Design review of the part shown in the three views and the two pictorial views. Dimensions are in mm from the part's minimum x, y and z. A direction names the side the tool comes from. Coordinates: 2 decimals unless noted, no trailing zeros. Loops run counter-clockwise (first coordinate to the right, second up) from the corner with the lowest first, then second, coordinate; pieces in that order, holes last. Notation, with made-up numbers: (37.25, 14) -> (54.25, 14) arc R27 ccw to (54.25, 52) -> close; hole circle Ø5 at (85, 69.25). An arc over 180 degrees is marked (long way). Answer in a Markdown table with one row per item.
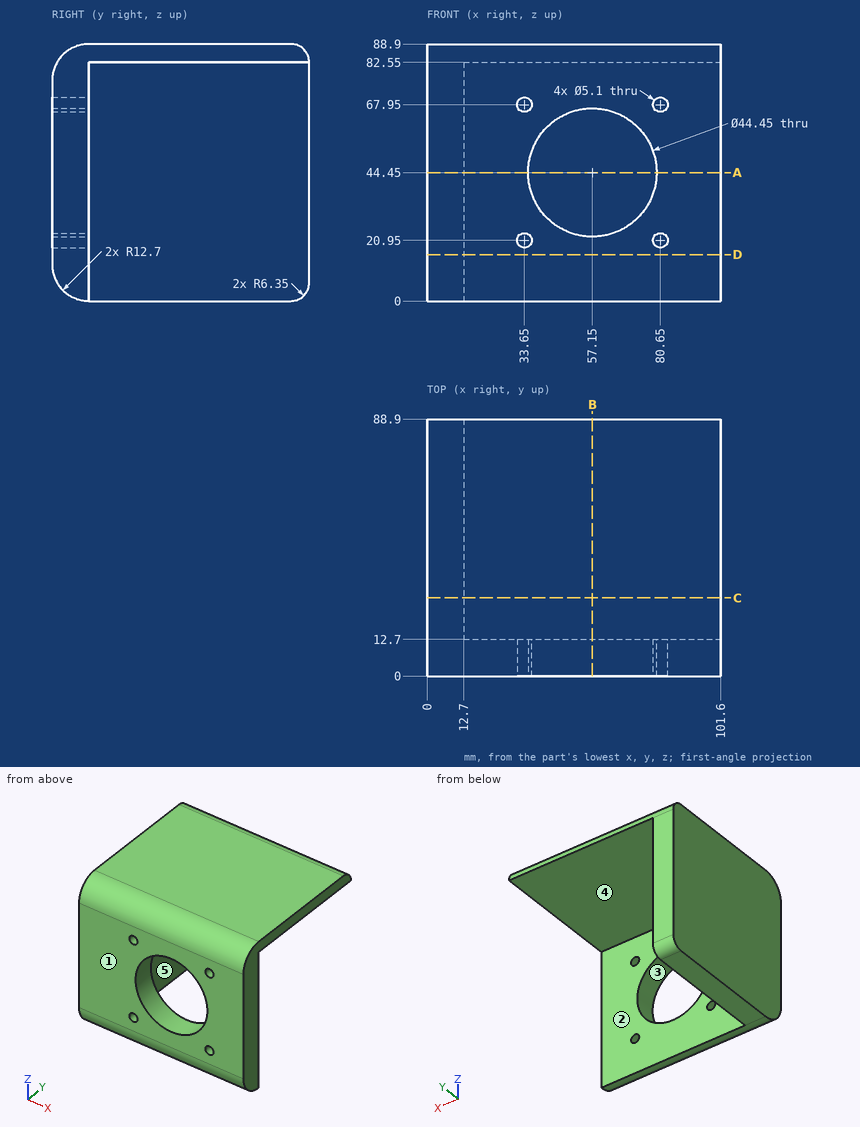
(1) Take a section at D-D on z = 16. Give the boundary of the cut face in (x, y).
Evaluation:
| item | result |
|---|---|
| outline | (0, 0) -> (101.6, 0) -> (101.6, 12.7) -> (12.7, 12.7) -> (12.7, 88.9) -> (0, 88.9) -> close |
(2) Take a section at C-C on y = 27. Give the boundary of the cut face in (x, z), and give its area (3 significant figures).
Evaluation:
| item | result |
|---|---|
| outline | (0, 0) -> (12.7, 0) -> (12.7, 82.55) -> (101.6, 82.55) -> (101.6, 88.9) -> (0, 88.9) -> close |
| area | 1,690 mm² |
(3) Tool access review of the marked faces 1 and 2: name each direction out of +Z, -Z, +X, -X, +Y, -Y from which nothing blocks a thin tool from reaching the whole face with its end or side.
Evaluation:
| item | result |
|---|---|
| face 1 | +Z, -Z, +X, -X, -Y |
| face 2 | -Z, +X, +Y |
(4) For pin 1 (6 mm diameter, centred on x = 38.5, z = 72.5, fed in from +Y); pin 2 (23 mm diameter, centred on y = 36.5, z = 55.5, fed in from +X); pin 3 (2 mm diameter, centred on x = 18, y = 77, fed in from -Z); pin 4 (4.5 mm diameter, centred on x = 80.65, z = 20.95, fed in from +Y), all flat-tipped, find the tip position at first contact; note any pin that passes through.
Evaluation:
| item | result |
|---|---|
| pin 1 | stops at y = 12.7 |
| pin 2 | stops at x = 12.7 |
| pin 3 | stops at z = 82.55 |
| pin 4 | passes through |
(5) Draft analysis for pull direction X (two halves, no side actions). For the marked faces 3, 4 and 5, state which applies: pulls with the +X half, pulls with the -X half, needs draft (parallel to the pull), parting line crosses it, or undercut.
Evaluation:
| item | result |
|---|---|
| face 3 | undercut |
| face 4 | needs draft |
| face 5 | pulls with the +X half |
(6) Take a section at A-A on z = 44.45. Give the boundary of the cut face in (x, y) (3 decimals).
Evaluation:
| item | result |
|---|---|
| outline | (0, 0) -> (34.925, 0) -> (34.925, 12.7) -> (12.7, 12.7) -> (12.7, 88.9) -> (0, 88.9) -> close; (79.375, 0) -> (101.6, 0) -> (101.6, 12.7) -> (79.375, 12.7) -> close |
(7) Take a section at B-B on x = 57.15. Give the boundary of the cut face in (y, z) (3 decimals), and give its area (3 significant figures).
Evaluation:
| item | result |
|---|---|
| outline | (0, 12.7) arc R12.7 ccw to (12.7, 0) -> (12.7, 22.225) -> (0, 22.225) -> close; (0, 66.675) -> (12.7, 66.675) -> (12.7, 82.55) -> (88.9, 82.55) arc R6.35 ccw to (82.55, 88.9) -> (12.7, 88.9) arc R12.7 ccw to (0, 76.2) -> close |
| area | 971 mm² |
(8) To check wall thickness, follow probe 1 along Z at (x, y) = (33.65, 4.75); probe 2 along Z at (x, y) = (33.65, 8.75); probe 3 along X at (y, z) = (34, 38). State the ranges of each line that lie inside material, in increasing order.
Evaluation:
| item | result |
|---|---|
| probe 1 | z = 2.8 to 18.4, 23.5 to 65.4, 70.5 to 86.1 |
| probe 2 | z = 0.63 to 18.4, 23.5 to 65.4, 70.5 to 88.27 |
| probe 3 | x = 0 to 12.7 |
